from build123d import *

# Parameters (mm, degrees)
SKETCH1_R           = 68.435
BOSS_EXTRUDE1_DEPTH = 415
BOSS_EXTRUDE1_TAPER = 4.4
SKETCH5_R           = 10
CUT_EXTRUDE1_DEPTH  = 10
CUT_EXTRUDE4_START  = 10
SKETCH4_R           = 10
CUT_EXTRUDE4_DEPTH  = 10
SKETCH9_R           = 10
BOSS_EXTRUDE2_DEPTH = 10
BOSS_EXTRUDE3_START = -10
SKETCH8_R           = 10
BOSS_EXTRUDE3_DEPTH = 10


with BuildPart() as part:
    # Sketch1 → Boss-Extrude1 (new body)
    with BuildSketch(Plane.XY):
        Circle(SKETCH1_R)
    extrude(amount=BOSS_EXTRUDE1_DEPTH, taper=BOSS_EXTRUDE1_TAPER)

    # Sketch2 → Revolve1 (revolve)
    with BuildSketch(Plane.XY.offset(415)):
        with BuildLine():
            Line((0, 31.50249031), (0, -31.50249031))
            ThreePointArc((0, -31.50249031), (-31.50249031, 0), (0, 31.50249031))
        make_face()
    revolve(axis=Axis((0, 31.50249031, 415), (0, -1, 0)))

    # Sketch3 → Cut-Revolve1 (revolve, cut)
    with BuildSketch(Plane(origin=(0, 0, 0), x_dir=(-1, 0, 0), z_dir=(0, 0, -1))):
        with BuildLine():
            Line((0, 63.435), (0, -63.435))
            ThreePointArc((0, -63.435), (-63.435, 0), (0, 63.435))
        make_face()
    revolve(axis=Axis((0, 63.435, 0), (0, -1, 0)), mode=Mode.SUBTRACT)

    # Sketch5 → Cut-Extrude1 (cut)
    with BuildSketch(Plane(origin=(-55, 0, 0), x_dir=(0, 0, -1), z_dir=(1, 0, 0))):
        with Locations((-16.443260801, 0)):
            Circle(SKETCH5_R)
    extrude(amount=-CUT_EXTRUDE1_DEPTH, mode=Mode.SUBTRACT)

    # Sketch4 → Cut-Extrude4 (cut)
    with BuildSketch(Plane(origin=(55, 0, 0), x_dir=(0, 0, -1), z_dir=(1, 0, 0)).offset(CUT_EXTRUDE4_START)):
        with Locations((-16.443260801, 0)):
            Circle(SKETCH4_R)
    extrude(amount=-CUT_EXTRUDE4_DEPTH, mode=Mode.SUBTRACT)

    # Sketch9 → Boss-Extrude2 (add)
    with BuildSketch(Plane(origin=(25, 0, 0), x_dir=(0, 0, -1), z_dir=(1, 0, 0))):
        with Locations(Location((-428.521516395, 0, 0), (0, 0, 108.224680934))):
            Circle(SKETCH9_R)
    extrude(amount=BOSS_EXTRUDE2_DEPTH)

    # Sketch8 → Boss-Extrude3 (add)
    with BuildSketch(Plane(origin=(-25, 0, 0), x_dir=(0, 0, -1), z_dir=(1, 0, 0)).offset(BOSS_EXTRUDE3_START)):
        with Locations(Location((-428.521516395, 0, 0), (0, 0, 108.224680934))):
            Circle(SKETCH8_R)
    extrude(amount=BOSS_EXTRUDE3_DEPTH)


solid = part.part
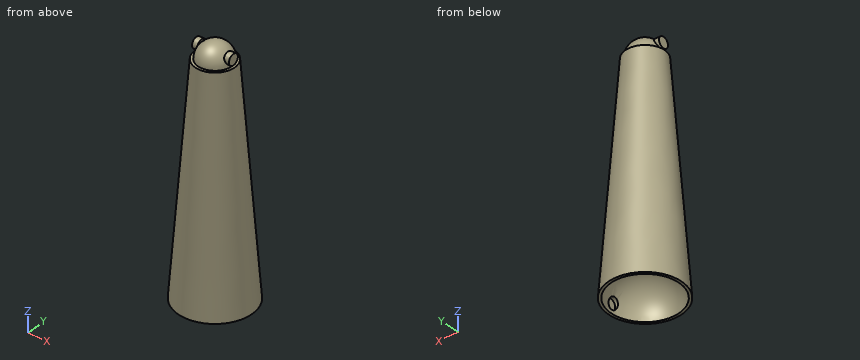
Read the model definition and answer for the solid it produces. Units are mm, in the model's axes. Round coordinates to 2 decimals unless told otherwise and drop trailing zeros. Order: outer loops, then holes, each group sorted by start corner. A loop starts at its lowest first (then second) coordinate and runs counter-clockwise, first axis right, second up.
1) The part is cut by section A-A on x = 0. Write down the section's boundary in (y, z) (1 decimal), plus the area to 3 significant figures.
2) The part is cut by section D-D on z = 248. Write down the section's boundary in (x, y).
3) The part is cut by section C-C on z = 120. Write down the section's boundary in (x, y), plus the area to 3 significant figures.
4) Straight lines are drawn through the part: L1, parallel to Y at x = 54, z = 19; L2, parallel to Y at x = -23.5, z = 51.5; L3, parallel to Y at x = -7.5, z = 316. For each, find the intervals that lie inside material, in ascending order.
5) Flat-ended cylindrical pins translate along their axes: pin 1 (12 mm diameter, centred on y = 0, z = 16.44, fed in from +X); pin 2 (4 mm diameter, centred on y = -24.5, z = 164, fed in from -X); pin 3 (10 mm diameter, centred on y = -37.5, z = 72.5, fed in from -X). Find the tip coordinate at first contact, or state that the pin passes through.
6) The part is cut by section B-B on y = 0. Write down the section's boundary in (x, z) (1 decimal), plus the area to 3 significant figures.
Resolved:
1. outline: (-68.4, 0) - (-63.4, 0) arc R63.4 cw to (63.4, 0) - (68.4, 0) - (36.5, 415) - (31.5, 415) arc R31.5 ccw to (-31.5, 415) - (-36.5, 415) - close
1. area: 38,800 mm2
2. outline: circle Ø98.7 at (0, 0)
3. outline: circle Ø118.4 at (0, 0)
3. area: 11,000 mm2
4. L1: y = -39.62 to -27.33, 27.33 to 39.62
4. L2: y = -60.04 to -28.63, 28.63 to 60.04
4. L3: y = -43.48 to 43.48
5. pin 1: stops at x = 67.63
5. pin 2: stops at x = -51.1
5. pin 3: stops at x = -53.84
6. outline: (-68.4, 0) - (-63.4, 0) arc R63.4 cw to (-63.1, 6.4) - (-65, 6.4) - (-65, 26.4) - (-57.7, 26.4) arc R63.4 cw to (57.7, 26.4) - (65, 26.4) - (65, 6.4) - (63.1, 6.4) arc R63.4 cw to (63.4, 0) - (68.4, 0) - (36.5, 415) - (31.5, 415) arc R31.5 ccw to (31.3, 418.5) - (35, 418.5) - (35, 438.5) - (25, 438.5) - (25, 434.2) arc R31.5 ccw to (-25, 434.2) - (-25, 438.5) - (-35, 438.5) - (-35, 418.5) - (-31.3, 418.5) arc R31.5 ccw to (-31.5, 415) - (-36.5, 415) - close
6. area: 38,900 mm2
